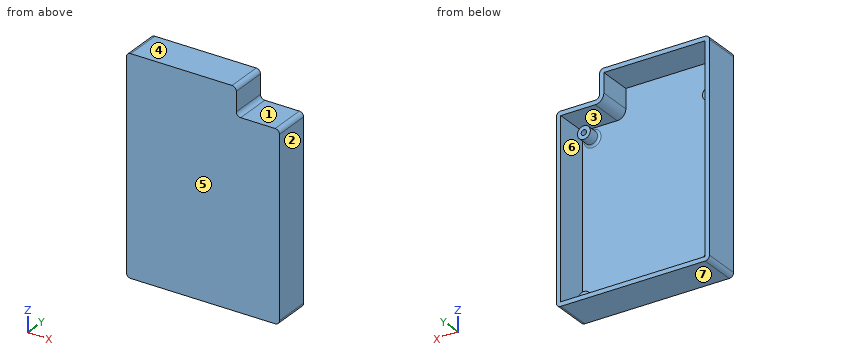
```python
from build123d import *

# Parameters (mm, degrees)
BOSS_EXTRUDE1_DEPTH = 1.5
SKETCH3_R           = 3
SKETCH3_R_2         = 1.25
BOSS_EXTRUDE3_DEPTH = 6
FILLET2_R           = 1
BOSS_EXTRUDE5_DEPTH = 15.5
FILLET6_R           = 2
FILLET7_R           = 4


with BuildPart() as part:
    # Sketch1 → Boss-Extrude1 (new body)
    with BuildSketch(Plane(origin=(0, 0, 0), x_dir=(1, 0, 0), z_dir=(0, 1, 0))):
        Polygon((35.5, 43), (-35.5, 43), (-35.5, -56), (15.5, -56), (15.5, -43), (35.5, -43), align=None)
    extrude(amount=BOSS_EXTRUDE1_DEPTH)

    # Sketch3 → Boss-Extrude3 (add)
    # profile 1 of 4: a face of its own
    with BuildSketch(Plane(origin=(0, 1.5, 0), x_dir=(1, 0, 0), z_dir=(0, 1, 0))):
        with Locations(Location((-29, 36.5, 0), (0, 0, 270))):
            Circle(SKETCH3_R)
        with Locations(Location((-29, 36.5, 0), (0, 0, 270))):
            Circle(SKETCH3_R_2, mode=Mode.SUBTRACT)
    # profile 2 of 4: a face of its own
    with BuildSketch(Plane(origin=(0, 1.5, 0), x_dir=(1, 0, 0), z_dir=(0, 1, 0))):
        with Locations(Location((29, 36.5, 0), (0, 0, 90))):
            Circle(SKETCH3_R)
        with Locations(Location((29, 36.5, 0), (0, 0, 90))):
            Circle(SKETCH3_R_2, mode=Mode.SUBTRACT)
    # profile 3 of 4: a face of its own
    with BuildSketch(Plane(origin=(0, 1.5, 0), x_dir=(1, 0, 0), z_dir=(0, 1, 0))):
        with Locations(Location((29, -36.5, 0), (0, 0, 270))):
            Circle(SKETCH3_R)
        with Locations(Location((29, -36.5, 0), (0, 0, 270))):
            Circle(SKETCH3_R_2, mode=Mode.SUBTRACT)
    # profile 4 of 4: a face of its own
    with BuildSketch(Plane(origin=(0, 1.5, 0), x_dir=(1, 0, 0), z_dir=(0, 1, 0))):
        with Locations(Location((-29, -36.5, 0), (0, 0, 90))):
            Circle(SKETCH3_R)
        with Locations(Location((-29, -36.5, 0), (0, 0, 90))):
            Circle(SKETCH3_R_2, mode=Mode.SUBTRACT)
    extrude(amount=BOSS_EXTRUDE3_DEPTH)

    # Fillet2
    fillet2_edges = [part.edges().sort_by_distance(p)[0] for p in [
        (-29, 1.5, -39.5),
        (29, 1.5, -33.5),
        (29, 1.5, 33.5),
        (-29, 1.5, 39.5),
    ]]
    fillet(fillet2_edges, radius=FILLET2_R)

    # Sketch5 → Boss-Extrude5 (add)
    with BuildSketch(Plane(origin=(0, 1.5, 0), x_dir=(1, 0, 0), z_dir=(0, 1, 0))):
        Polygon((-35.5, 43), (-35.5, -56), (15.5, -56), (15.5, -43), (35.5, -43), (35.5, 43), align=None)
        Polygon((-33.5, 41), (-33.5, -54), (13.5, -54), (13.5, -41), (33.5, -41), (33.5, 41), align=None, mode=Mode.SUBTRACT)
    extrude(amount=BOSS_EXTRUDE5_DEPTH)

    # Fillet6
    fillet6_edges = [part.edges().sort_by_distance(p)[0] for p in [
        (-35.5, 8.5, -43),
        (35.5, 8.5, -43),
        (35.5, 8.5, 43),
        (15.5, 8.5, 43),
        (15.5, 8.5, 56),
        (-35.5, 8.5, 56),
    ]]
    fillet(fillet6_edges, radius=FILLET6_R)

    # Fillet7
    fillet7_edges = [part.edges().sort_by_distance(p)[0] for p in [
        (13.5, 9.25, 41),
    ]]
    fillet(fillet7_edges, radius=FILLET7_R)


solid = part.part
```
Input: part model. Units: mm. Frame: model coordinates. Face numbers are marked on the shaded views. A direction names the side the tool comes from. Coordinates: 2 decimals unless noted, no trailing zeros. Write each loop counter-clockwise with the first axis right and the second up, starting at its lowest first coordinate (ties: lowest second). Pieces come first, ordered by that corner, then holes. Notation, with made-up numbers: (6.25, 70) -> (19.25, 70) arc R22 cw to (19.25, 78) -> close; hole circle Ø9 at (55.5, 11). An arc over 180 degrees is marked (long way). Write each question's results on one line, items separated by ' | '.
Item 1: Section query C-C on x = 29. Return loops of the section in (y, z), plus the area to 3 significant figures.
Conclusion:
outline: (0, -43) -> (17, -43) -> (17, -41) -> (1.5, -41) -> (1.5, -40.5) arc R1 cw to (2.5, -39.5) -> (7.5, -39.5) -> (7.5, -37.75) -> (1.5, -37.75) -> (1.5, -35.25) -> (7.5, -35.25) -> (7.5, -33.5) -> (2.5, -33.5) arc R1 cw to (1.5, -32.5) -> (1.5, 32.5) arc R1 cw to (2.5, 33.5) -> (7.5, 33.5) -> (7.5, 35.25) -> (1.5, 35.25) -> (1.5, 37.75) -> (7.5, 37.75) -> (7.5, 39.5) -> (2.5, 39.5) arc R1 cw to (1.5, 40.5) -> (1.5, 41) -> (17, 41) -> (17, 43) -> (0, 43) -> close | area: 234 mm^2
Item 2: Section query A-A on y = 6. Count the separate pieces of the cut face and the enclosed holes in it, plus the area to 3 significant figures.
Conclusion:
separate pieces: 5 | enclosed holes: 5 | area: 751 mm^2
Item 3: Set-up query: the marked faces 1, 2 and 3. Return all of +Z, -Z, +X, -X, +Y, -Y with unobstructed straight access to the full face (end or side cutting, diameter ignored); none if empty.
Conclusion:
face 1: +Z, +X, +Y, -Y | face 2: +Z, -Z, +X, +Y, -Y | face 3: +Y
Item 4: Section query B-B on y = 16. Return loops of the section in (x, z).
Conclusion:
outline: (-35.5, -41) arc R2 ccw to (-33.5, -43) -> (33.5, -43) arc R2 ccw to (35.5, -41) -> (35.5, 41) arc R2 ccw to (33.5, 43) -> (17.5, 43) arc R2 cw to (15.5, 45) -> (15.5, 54) arc R2 ccw to (13.5, 56) -> (-33.5, 56) arc R2 ccw to (-35.5, 54) -> close; hole (-33.5, -41) -> (33.5, -41) -> (33.5, 41) -> (17.5, 41) arc R4 cw to (13.5, 45) -> (13.5, 54) -> (-33.5, 54) -> close
Item 5: Pin query (flat end, axial travel): pin 1 Ø1.8 at (x, z) = (-28.5, -36.5) entering from +Y; pin 2 Ø2 at (x, z) = (-29, -36.5) entering from +Y; pin 3 Ø1.5 at (x, z) = (-15, -31) entering from -Y. Return the tip coordinate at first contact, or that it passes through.
Conclusion:
pin 1: stops at y = 7.5 | pin 2: stops at y = 1.5 | pin 3: stops at y = 0
Item 6: Material intervals for probe 1 along X at (y, z) = (5.2, 36.5); probe 2 along Z at (x, y) = (10.5, 13.5); probe 3 along X at (y, z) = (8, -18), sorted ascending.
Conclusion:
probe 1: x = -35.5 to -33.5, -32 to -30.25, -27.75 to -26, 26 to 27.75, 30.25 to 32, 33.5 to 35.5 | probe 2: z = -43 to -41, 54 to 56 | probe 3: x = -35.5 to -33.5, 33.5 to 35.5
Item 7: Mould query, pull axis Z, two halves, no side actions, for the marked faces 4, 5, 6 and 7. Classes: +Z half, -Z half, draft (parallel to the pull), parting line (faces both ways), or undercut.
Conclusion:
face 4: +Z half | face 5: draft | face 6: undercut | face 7: -Z half
Item 8: Section query D-D on z = 48. Return loops of the section in (x, y), plus the area to 4 significant figures.
Conclusion:
outline: (-35.5, 0) -> (15.5, 0) -> (15.5, 17) -> (13.5, 17) -> (13.5, 1.5) -> (-33.5, 1.5) -> (-33.5, 17) -> (-35.5, 17) -> close | area: 138.5 mm^2
